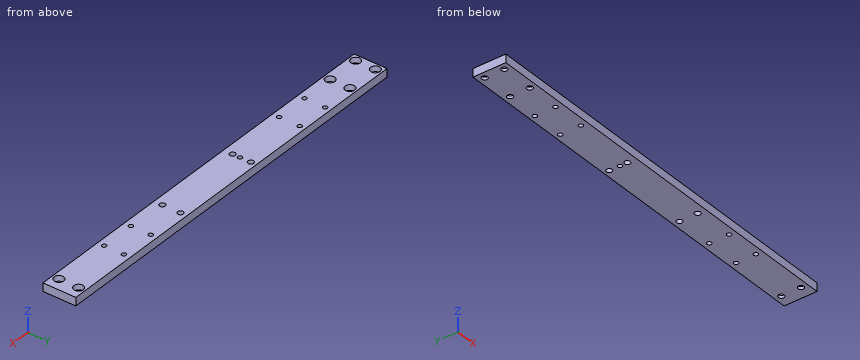
from build123d import *

# Parameters (mm, degrees)
F0_W     = 465.86
F0_H     = 38.1
F0_R     = 3.38
F0_R_2   = 2.555
F0_R_3   = 3.3
F1_DEPTH = 9.53
F2_R     = 5.555
F3_DEPTH = 6.35


with BuildPart() as f1:
    # F0 (on Top) → F1 (new body)
    with BuildSketch(Plane.XY):
        with Locations((-291.849708, -205.635505)):
            Rectangle(F0_W, F0_H)
        with Locations((-517.159708, -217.065505)):
            Circle(F0_R, mode=Mode.SUBTRACT)
        with Locations((-479.059708, -217.065505)):
            Circle(F0_R, mode=Mode.SUBTRACT)
        with Locations((-440.599708, -217.065505)):
            Circle(F0_R_2, mode=Mode.SUBTRACT)
        with Locations((-402.499708, -217.065505)):
            Circle(F0_R_2, mode=Mode.SUBTRACT)
        with Locations((-329.269708, -214.155505)):
            Circle(F0_R_3, mode=Mode.SUBTRACT)
        with Locations((-180.689708, -217.065505)):
            Circle(F0_R_2, mode=Mode.SUBTRACT)
        with Locations((-140.589708, -217.065505)):
            Circle(F0_R_2, mode=Mode.SUBTRACT)
        with Locations((-72.899708, -217.065505)):
            Circle(F0_R, mode=Mode.SUBTRACT)
        with Locations((-225.289708, -215.155505)):
            Circle(F0_R_3, mode=Mode.SUBTRACT)
        with Locations((-329.269708, -205.635505)):
            Circle(F0_R_2, mode=Mode.SUBTRACT)
        with Locations((-517.159708, -194.205505)):
            Circle(F0_R, mode=Mode.SUBTRACT)
        with Locations((-479.059708, -194.205505)):
            Circle(F0_R, mode=Mode.SUBTRACT)
        with Locations((-440.599708, -193.105505)):
            Circle(F0_R_2, mode=Mode.SUBTRACT)
        with Locations((-402.499708, -193.105505)):
            Circle(F0_R_2, mode=Mode.SUBTRACT)
        with Locations((-329.269708, -193.105505)):
            Circle(F0_R_3, mode=Mode.SUBTRACT)
        with Locations((-225.289708, -194.105505)):
            Circle(F0_R_3, mode=Mode.SUBTRACT)
        with Locations((-180.689708, -194.105505)):
            Circle(F0_R_2, mode=Mode.SUBTRACT)
        with Locations((-140.589708, -194.205505)):
            Circle(F0_R_2, mode=Mode.SUBTRACT)
        with Locations((-72.899708, -194.205505)):
            Circle(F0_R, mode=Mode.SUBTRACT)
    extrude(amount=F1_DEPTH)

    # F2 (on face) → F3 (cut)
    with BuildSketch(Plane.XY.offset(9.53)):
        with Locations((-517.159708, -194.205505)):
            Circle(F2_R)
        with Locations((-517.159708, -217.065505)):
            Circle(F2_R)
        with Locations((-479.059708, -194.205505)):
            Circle(F2_R)
        with Locations((-479.059708, -217.065505)):
            Circle(F2_R)
        with Locations((-72.899708, -194.205505)):
            Circle(F2_R)
        with Locations((-72.899708, -217.065505)):
            Circle(F2_R)
    extrude(amount=-F3_DEPTH, mode=Mode.SUBTRACT)


solid = f1.part
The model under review builds one solid part; all positions refer to its coordinate system, in mm. Give positions to 0.01 mm unless a question says otherwise; leave off trailing zeros. Put each result on its own line as item: value. Start each with the question number.
1. We need section A-A on z = 6. State how many separate pieces and enclosed holes the cut face has, then the cut area to 3 significant figures.
2. Wall thickness on probe 1 along X at (y, z) = (-221.5, 3.25); probe 2 along X at (y, z) = (-197.5, 4); probe 3 along X at (y, z) = (-211.5, 2): over which ranges is each line inside the solid? List them lowest first.
3. Clearance check with flat-ended pins moving along their axes: P1, Ø12, axis at x = -75, y = -219, coming from the +Z side; P2, Ø8, axis at x = -479.06, y = -194.21, coming from the +Z side. State where each tip first meets the part, or that it passes through.
Determined:
1. separate pieces: 1
1. enclosed holes: 19
1. area: 16,800 mm^2
2. probe 1: -524.78 to -520.51, -513.81 to -482.41, -475.71 to -76.25, -69.55 to -58.92
2. probe 2: -524.78 to -521.63, -512.69 to -483.53, -474.59 to -77.37, -68.43 to -58.92
2. probe 3: -524.78 to -331.23, -327.31 to -58.92
3. P1: z = 9.53
3. P2: z = 3.18
